Model file for the job. Use its own axes, mm. A direction names the side the tool comes from. Round coordinates to 2 decimals unless told otherwise and drop trailing zeros. Loops run counter-clockwise (first coordinate to the right, second up) from the corner with the lowest first, then second, coordinate; pieces in that order, holes last.
Autodesk Inventor part; units mm, degrees
ref_plane "YZ Plane" through (0, 0, 0) normal (1, 0, 0) x (0, 1, 0)
ref_plane "XZ Plane" through (0, 0, 0) normal (0, 1, 0) x (-1, 0, 0)
ref_plane "XY Plane" through (0, 0, 0) normal (0, 0, 1) x (1, 0, 0)
sketch "Sketch1" plane through (0, 0, 0) normal (0, 0, 1) x (1, 0, 0)
  line L0 (-22.0262, 11.1206) -> (35.1238, 11.1206)
  line L1 (35.1238, 11.1206) -> (35.1238, -20.6294)
  line L2 (35.1238, -20.6294) -> (-22.0262, -20.6294)
  line L3 (-22.0262, -20.6294) -> (-22.0262, 11.1206)
  point P0 (0, 0)
  dimension "d0" = 57.15
  dimension "d1" = 31.75
extrude "Extrusion1" add sketch "Sketch1" along normal blind 31.75
sketch "Sketch2" plane through (0, 0, 31.75) normal (0, 0, 1) x (1, 0, 0)
  line L0 (35.1238, 11.1206) -> (-22.0262, 11.1206)
  line L1 (-22.0262, 11.1206) -> (35.1238, 11.1206)
  line L2 (35.1238, 11.1206) -> (35.1238, -7.9294)
  line L3 (35.1238, -7.9294) -> (-22.0262, -7.9294)
  line L4 (-22.0262, -7.9294) -> (-22.0262, 11.1206)
  point P0 (0, 0)
  dimension "d4" = 19.05
  dimension "d5" = 57.15
extrude "Extrusion2" cut sketch "Sketch2" against normal blind 19.05
sketch "Sketch3" plane through (0, 0, 31.75) normal (0, 0, 1) x (1, 0, 0)
  line L0 (-22.0262, -20.6294) -> (35.1238, -20.6294)
  line L1 (35.1238, -20.6294) -> (22.4238, -7.9294)
  line L2 (35.1238, -7.9294) -> (-22.0262, -7.9294)
  line L3 (22.4238, -7.9294) -> (35.1238, -7.9294)
  line L4 (35.1238, 11.1206) -> (35.1238, -20.6294)
  line L5 (35.1238, -7.9294) -> (35.1238, -20.6294)
  point P0 (0, 0)
  dimension "d8" = 44.45
extrude "Extrusion3" cut sketch "Sketch3" against normal blind 19.05
sketch "Sketch4" plane through (0, 0, 0) normal (0, 0, -1) x (-1, 0, 0)
  line L0 (-35.1238, -20.6294) -> (-22.4238, -7.9294)
  line L1 (-35.1238, -20.6294) -> (-3.3738, 11.1206)
  line L2 (22.0262, 11.1206) -> (-35.1238, 11.1206)
  line L3 (-3.3738, 11.1206) -> (-35.1238, 11.1206)
  line L4 (-35.1238, 11.1206) -> (-35.1238, -20.6294)
  line L5 (-35.1238, 11.1206) -> (-35.1238, -20.6294)
  point P0 (0, 0)
  dimension "d11" = 25.4
extrude "Extrusion4" cut sketch "Sketch4" against normal blind 19.05
properties part number "Figure 7_28_6"
Q1. Tool access for faces 1 (the face through (0, -8, 0)), 2 (the face through (1, -7.929, 22)): list every direction of +Z, -Z, +X, -X, +Y, -Y with a clear straight run to the whole face (end or side of a thin tool).
Q2. Slice it at A-A on x = -4. Give the cut face in (y, z), plus the area to 3 significant figures.
Q3. Slice it at D-D on x = 8. Give the cut face in (y, z).
Q4. Probe line 1 (Z direction, x = -2.5, y = -4.5); line 2 (Y direction, x = -13, z = 17.5); line 3 (X direction, y = -9, z = 30). List the from-to ranges inside material, lowest first.
Q5. Slice it at B-B on z = 28.5. Give the cut face in (x, y).
Q6. Slice it at C-C on y = -3.5. Give the cut face in (x, z).
Q7. Flat gauge pins, fed straight in: P1, Ø9.5, axis at x = -6.5, y = 2.5, coming from the +Z side; P2, Ø9.5, axis at x = -5, z = 25.5, coming from the +Y side. Where does each tip first touch, or does it go through?
Reply:
1. face 1: -Z, +X, -X, +Y, -Y
1. face 2: +Z, +X, -X, +Y
2. outline: (-20.63, 0) - (11.12, 0) - (11.12, 12.7) - (-7.93, 12.7) - (-7.93, 31.75) - (-20.63, 31.75) - close
2. area: 645 mm2
3. outline: (-20.63, 0) - (6.49, 0) - (6.49, 12.7) - (-7.93, 12.7) - (-7.93, 31.75) - (-20.63, 31.75) - close
4. line 1: z = 0 to 12.7
4. line 2: y = -20.63 to -7.93
4. line 3: x = -22.03 to 23.49
5. outline: (-22.03, -20.63) - (35.12, -20.63) - (22.42, -7.93) - (-22.03, -7.93) - close
6. outline: (-22.03, 0) - (17.99, 0) - (17.99, 12.7) - (-22.03, 12.7) - close
7. P1: stops at z = 12.7
7. P2: stops at y = -7.93
